The listing builds one solid part. Answer for the finished solid, in the listing's coordinates (mm). Give positions to 0.01 mm unless a question says otherwise; leave off trailing zeros. Loops run counter-clockwise (first coordinate to the right, second up) from the corner with the lowest first, then second, coordinate; pieces in that order, holes last. Notation, with made-up numbers: (51.25, -27) -> (67.25, -27) arc R16 cw to (67.25, -19) -> close; hole circle Ø6 at (23.5, 19). An arc over 180 degrees is marked (long way). One line per question, with ' | ' between items. Start each with the question number.
Autodesk Inventor part; units mm, degrees
ref_plane "YZ Plane" through (0, 0, 0) normal (1, 0, 0) x (0, 1, 0)
ref_plane "XZ Plane" through (0, 0, 0) normal (0, 1, 0) x (-1, 0, 0)
ref_plane "XY Plane" through (0, 0, 0) normal (0, 0, 1) x (1, 0, 0)
sketch "스케치3" plane through (0, 0, 0) normal (0, 0, 1) x (1, 0, 0)
  line L0 (-232, 158) -> (232, 158)
  line L1 (232, 158) -> (232, -158)
  line L2 (232, -158) -> (-232, -158)
  line L3 (-232, -158) -> (-232, 158)
  line L4 (-212, -9.5) -> (-83.5, -9.5)
  line L5 (-83.5, -9.5) -> (-83.5, -138)
  line L6 (-83.5, -138) -> (-212, -138)
  line L7 (-212, -138) -> (-212, -9.5)
  line L8 (-212, 138) -> (-83.5, 138)
  line L9 (-83.5, 138) -> (-83.5, 9.5)
  line L10 (-83.5, 9.5) -> (-212, 9.5)
  line L11 (-212, 9.5) -> (-212, 138)
  line L12 (212, 138) -> (83.5, 138)
  line L13 (83.5, 138) -> (83.5, 9.5)
  line L14 (83.5, 9.5) -> (212, 9.5)
  line L15 (212, 9.5) -> (212, 138)
  line L16 (212, -138) -> (83.5, -138)
  line L17 (83.5, -138) -> (83.5, -9.5)
  line L18 (83.5, -9.5) -> (212, -9.5)
  line L19 (212, -9.5) -> (212, -138)
  circle A0 centre (-42.072, 42.072) radius 2
  circle A1 centre (42.072, 42.072) radius 2
  circle A2 centre (-42.072, -42.072) radius 2
  circle A3 centre (42.072, -42.072) radius 2
  line L20 (0, -221.2) -> (0, 221.2)
  line L21 (-324.8, 0) -> (324.8, 0)
  circle A4 centre (0, 0) radius 50
  point P0 (232, 0)
  point P1 (212, 73.75)
  dimension "d0" = 316
  dimension "d1" = 464
  dimension "d2" = 232
  dimension "d3" = 158
  dimension "d4" = 128.5
  dimension "d5" = 128.5
  dimension "d6" = 20
  dimension "d7" = 20
  dimension "d8" = 128.5
  dimension "d9" = 128.5
  dimension "d10" = 20
  dimension "d11" = 20
  dimension "d12" = 128.5
  dimension "d13" = 128.5
  dimension "d14" = 20
  dimension "d15" = 128.5
  dimension "d16" = 128.5
  dimension "d17" = 20
  dimension "d18" = 20
  dimension "d19" = 4
  dimension "d20" = 4
  dimension "d21" = 4
  dimension "d22" = 4
  dimension "d23" = 42.072
  dimension "d24" = 42.072
  dimension "d25" = 42.072
  dimension "d26" = 42.072
  dimension "d27" = 42.072
  dimension "d28" = 42.072
  dimension "d29" = 42.072
  dimension "d30" = 42.072
  dimension "d31" = 100
extrude "돌출1" add sketch "스케치3" along normal blind 5 contours L0 L20 A4 L21 L3 | L0 L1 L21 A4 L20 | L21 A4 L20 L2 L3 | L1 L2 L20 A4 L21
properties part number "가로세로"
1. The part is cut by section B-B (y = 0). Write down the section's boundary in (x, z), plus the area to 3 significant figures.
2. Straight lines are drawn through the part: L1, parallel to Y at x = -122, z = 4.6; L2, parallel to X at y = 61, z = 3.45; L3, parallel to Y at x = 0, z = 1.55. For each, find the intervals that lie inside material, in ascending order.
3. Each of these flat-tipped pins is pushed along its axis until it touches: pin 1 Ø3 at (x, y) = (-42.072, -42.072) entering from -Z (3 decimals); pin 2 Ø5 at (x, y) = (40, 48) entering from -Z. Where does it stop, or does it pass through?
4. The part is cut by section C-C (x = 194). Write down the section's boundary in (y, z).
5. The part is cut by section A-A (x = 0). Write down the section's boundary in (y, z), plus the area to 3 significant figures.
6. Determine the mould class of faces 1 (the cylindrical face through (47.69, -15.02, 2.46)), 2 (the flat face through (-55, 2, 0)) for opening direction X: released by +X, released by -X, zero draft, split by the parting line, or undercut.
Check sheet entries:
1) outline: (-232, 0) -> (-50, 0) -> (-50, 5) -> (-232, 5) -> close; (50, 0) -> (232, 0) -> (232, 5) -> (50, 5) -> close | area: 1,820 mm^2
2) L1: y = -158 to -138, -9.5 to 9.5, 138 to 158 | L2: x = -232 to -212, -83.5 to 83.5, 212 to 232 | L3: y = -158 to -50, 50 to 158
3) pin 1: passes through | pin 2: stops at z = 0
4) outline: (-158, 0) -> (-138, 0) -> (-138, 5) -> (-158, 5) -> close; (-9.5, 0) -> (9.5, 0) -> (9.5, 5) -> (-9.5, 5) -> close; (138, 0) -> (158, 0) -> (158, 5) -> (138, 5) -> close
5) outline: (-158, 0) -> (-50, 0) -> (-50, 5) -> (-158, 5) -> close; (50, 0) -> (158, 0) -> (158, 5) -> (50, 5) -> close | area: 1,080 mm^2
6) face 1: undercut | face 2: zero draft
